Job drawing, mm, ordinate dimensions from the low corner. One solid piece. Coordinates: 2 decimals unless noted, no trailing zeros. Write each loop counter-clockwise with the first axis right and the second up, starting at its lowest first coordinate (ties: lowest second). Pieces come first, ordered by that corner, then holes. Notation, with made-up numbers: (-35.5, 19) - (23.5, 19) arc R26 ccw to (23.5, 49) - close; hole circle Ø9 at (-37, 39). An arc over 180 degrees is marked (long way). Use one line per item in the form item = value. Start each with the question number.
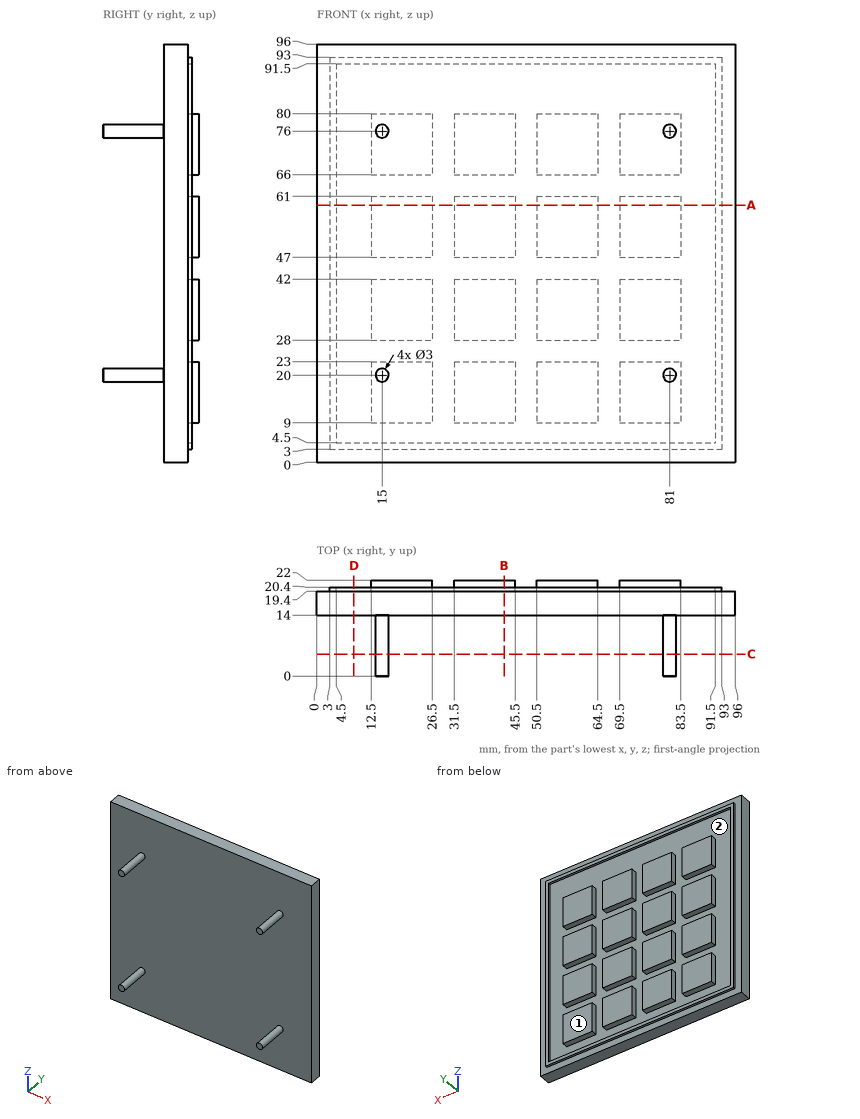
Q1. Slice it at B-B (x = 43). List the corners of the cut face in (y, z), plus the area to 3 significant figures.
Q2. Slice it at A-A (z = 59). List the corners of the cut face in (x, y), plus the area to 3 significant figures.
Q3. Slice it at C-C (y = 5). List the corners of the cut face in (x, z), plus the area to 3 significant figures.
Q4. Mould opens along Z. For the marked faces 1 and 2 say: released by +Z, released by -Z, zero draft, split by the parting line, or undercut.
Q5. Drill centre lines: probe 1 along Z at (x, y) = (52, 19.5); probe 2 along X at (y, z) = (21, 50); probe 3 along Z at (x, y) = (48, 20). Where is each one in solid material? Low to high.
Q6. Slice it at D-D (x = 8.5). List the corners of the cut face in (y, z), plus the area to 3 significant figures.
Q7. Pin check, flat tips, straight feed: P1, Ø0.8, axis at y = 20, z = 16.5, coming from the -X side; P2, Ø10, axis at x = 9.5, y = 13.5, coming from the +Z side; P3, Ø0.8, axis at x = 17.5, y = 20, coming from the -Z side; P4, Ø0.8, axis at x = 55, y = 21, coming from the +Z side. Stop position of each tip, or through.
Solution:
q1.outline = (14, 0) - (19.4, 0) - (19.4, 3) - (20.4, 3) - (20.4, 4.5) - (19.4, 4.5) - (19.4, 9) - (22, 9) - (22, 23) - (19.4, 23) - (19.4, 28) - (22, 28) - (22, 42) - (19.4, 42) - (19.4, 47) - (22, 47) - (22, 61) - (19.4, 61) - (19.4, 66) - (22, 66) - (22, 80) - (19.4, 80) - (19.4, 91.5) - (20.4, 91.5) - (20.4, 93) - (19.4, 93) - (19.4, 96) - (14, 96) - close
q1.area = 667 mm2
q2.outline = (0, 14) - (96, 14) - (96, 19.4) - (93, 19.4) - (93, 20.4) - (91.5, 20.4) - (91.5, 19.4) - (83.5, 19.4) - (83.5, 22) - (69.5, 22) - (69.5, 19.4) - (64.5, 19.4) - (64.5, 22) - (50.5, 22) - (50.5, 19.4) - (45.5, 19.4) - (45.5, 22) - (31.5, 22) - (31.5, 19.4) - (26.5, 19.4) - (26.5, 22) - (12.5, 22) - (12.5, 19.4) - (4.5, 19.4) - (4.5, 20.4) - (3, 20.4) - (3, 19.4) - (0, 19.4) - close
q2.area = 667 mm2
q3.outline = circle Ø3 at (15, 20); circle Ø3 at (15, 76); circle Ø3 at (81, 20); circle Ø3 at (81, 76)
q3.area = 28.3 mm2
q4.face_1 = zero draft
q4.face_2 = undercut
q5.probe_1 = 3 to 4.5, 9 to 23, 28 to 42, 47 to 61, 66 to 80, 91.5 to 93
q5.probe_2 = 12.5 to 26.5, 31.5 to 45.5, 50.5 to 64.5, 69.5 to 83.5
q5.probe_3 = 3 to 4.5, 91.5 to 93
q6.outline = (14, 0) - (19.4, 0) - (19.4, 3) - (20.4, 3) - (20.4, 4.5) - (19.4, 4.5) - (19.4, 91.5) - (20.4, 91.5) - (20.4, 93) - (19.4, 93) - (19.4, 96) - (14, 96) - close
q6.area = 521 mm2
q7.P1 = 3
q7.P2 = 96
q7.P3 = 3
q7.P4 = 80
